Solid Edge part; units mm, degrees
sketch "Sketch1" plane through (0, 0, 0) normal (1, 0, 0) x (0, 1, 0)
  line L0 (-4, 4) -> (-4, 23)
  line L1 (-4, 23) -> (0, 23)
  line L2 (0, 23) -> (0, 0)
  line L3 (0, 0) -> (-23, 0)
  line L4 (-23, 0) -> (-23, 4)
  line L5 (-23, 4) -> (-4, 4)
extrude "Protrusion1" add sketch "Sketch1" along normal mid plane 38
hole "Agujero_1" at (10, -4, 15) direction (0, 1, 0) diameter 3.2 end up to next
hole "Hole1" at (-10, -4, 15) direction (0, 1, 0) diameter 3.2 end up to next
hole "Agujero_3" at (10, -15, 4) direction (0, 0, -1) diameter 3.2 end up to next
hole "Hole2" at (-10, -15, 4) direction (0, 0, -1) diameter 3.2 end up to next
Read the model definition and answer for the solid it produces. Units are mm, in the model's axes. A direction names the side the tool comes from. Give positions to 0.01 mm unless a question says otherwise; leave off trailing zeros. Write each loop counter-clockwise with the first axis right and the second up, starting at its lowest first coordinate (ties: lowest second). Pieces come first, ordered by that corner, then holes. Notation, with made-up numbers: (10.25, -21.75) -> (46.25, -21.75) arc R11 ccw to (46.25, -1.75) -> close; hole circle Ø1 at (-15.5, 24). An arc over 180 degrees is marked (long way). Answer as a JSON object with one key per item and string values. Group by question number.
1) A tool of negligible diameter and unlimited length cuts with its end or side. For faces 1 (the flat face through (0, -4, 13)), 2 (the flat face through (0, -23, 2)), from which of +Z, -Z, +X, -X, +Y, -Y can it reach the whole face along a straight path? Write none if from no direction.
2) The mould has two halves that part along X. Classify faces 3 (the cylindrical face through (-10.97, -13.73, 2.03)), 4 (the flat face through (0, -14, 4)): +X half, -X half, draft (parallel to the pull), parting line (faces both ways), or undercut.
3) Find section A-A (y = -15). Write down the section's boundary in (x, z), and give its area (3 significant figures).
4) Find section C-C (z = 15). Write down the section's boundary in (x, y), and give its area (3 significant figures).
5) Find section D-D (y = -2.5). Write down the section's boundary in (x, z), and give its area (3 significant figures).
6) Consider L1, parallel to X at y = -15, z = 2.75; L2, parallel to Z at x = 10, y = -1; L3, parallel to Y at x = 10, z = 1.5. Determine where each line is inside the solid, lowest interval first. Write a range as from..to.
7) Each of these flat-tipped pins is pushed along its axis until it touches: P1, Ø5.5, axis at x = -8, z = 13, coming from the -Y side; P2, Ø9.5, axis at x = 1, y = -15, coming from the +Z side. Where does it stop, or does it pass through?
8) Find section B-B (x = -10). Write down the section's boundary in (y, z).
Values follow:
{
 "1": {"face 1": "+Z, +X, -X, -Y", "face 2": "+Z, -Z, +X, -X, -Y"},
 "2": {"face 3": "undercut", "face 4": "draft"},
 "3": {"outline": "(-19, 0) -> (-11.6, 0) -> (-11.6, 4) -> (-19, 4) -> close; (-8.4, 0) -> (8.4, 0) -> (8.4, 4) -> (-8.4, 4) -> close; (11.6, 0) -> (19, 0) -> (19, 4) -> (11.6, 4) -> close", "area": "126 mm2"},
 "4": {"outline": "(-19, -4) -> (-11.6, -4) -> (-11.6, 0) -> (-19, 0) -> close; (-8.4, -4) -> (8.4, -4) -> (8.4, 0) -> (-8.4, 0) -> close; (11.6, -4) -> (19, -4) -> (19, 0) -> (11.6, 0) -> close", "area": "126 mm2"},
 "5": {"outline": "(-19, 0) -> (19, 0) -> (19, 23) -> (-19, 23) -> close; hole circle Ø3.2 at (-10, 15); hole circle Ø3.2 at (10, 15)", "area": "858 mm2"},
 "6": {"L1": "x = -19..-11.6, -8.4..8.4, 11.6..19", "L2": "z = 0..13.4, 16.6..23", "L3": "y = -23..-16.6, -13.4..0"},
 "7": {"P1": "stops at y = -4", "P2": "stops at z = 4"},
 "8": {"outline": "(-23, 0) -> (-16.6, 0) -> (-16.6, 4) -> (-23, 4) -> close; (-13.4, 0) -> (0, 0) -> (0, 13.4) -> (-4, 13.4) -> (-4, 4) -> (-13.4, 4) -> close; (-4, 16.6) -> (0, 16.6) -> (0, 23) -> (-4, 23) -> close"}
}
